The figure shows three views and two pictorial views of one solid part (mm, origin at its lowest corner). Answer the questions. Round coordinates to 2 decimals unless told otherwise and drop trailing zeros. Write each loop counter-clockwise with the first axis right and the second up, starting at its lowest first coordinate (ties: lowest second). Pieces come first, ordered by that corner, then holes. Notation, with made-up numbers: M 15.25,24 L 45.25,24 A11 cw 45.25,45 Z; hole C -17.75,6 d11. An arc over 180 degrees is marked long. One line per item, written item: value. Start each with the question number.
Q1. Consider probe 1 along X at (y, z) = (2.75, 5); probe 2 along Y at (x, z) = (22, 2.75); probe 3 along X at (y, z) = (20.25, 8.25). Determine where each line is inside the solid, lowest interval first.
Q2. The mould has two halves that part along Y. Classify the marked faces 1, 2 and 3: released by +Y, released by -Y, zero draft, split by the parting line, or undercut.
Q3. Find section D-D (x = 8). Write down the section's boundary in (y, z).
Q4. Find section B-B (y = 16.5). Write down the section's boundary in (x, z), and give its area (3 significant figures).
Q5. Find section C-C (z = 1.25). Write down the section's boundary in (x, y), and give its area (3 significant figures).
Q6. Given pin 1 Ø1.5 at (x, z) = (7.5, 6) entering from -Y, flat-ended and moving along its own axis, determine where the tip first touches the part or whether it passes through.
Q7. Find section A-A (x = 75.98). Write down the section's boundary in (y, z), and give its area (3 significant figures).
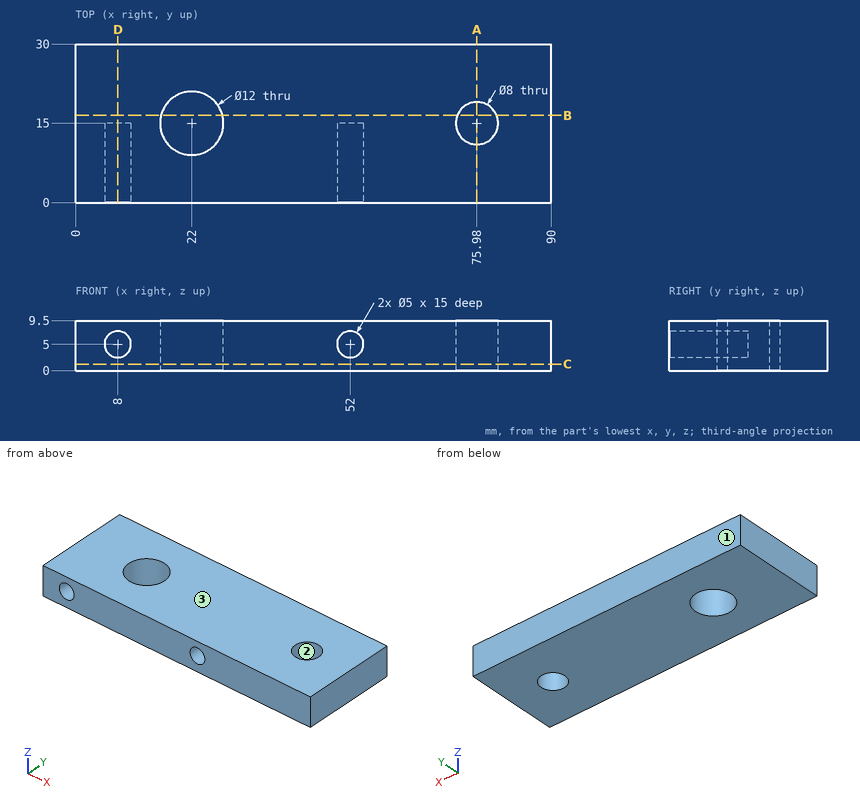
The answers:
1. probe 1: 0 to 5.5, 10.5 to 49.5, 54.5 to 90
1. probe 2: 0 to 9, 21 to 30
1. probe 3: 0 to 19.1, 24.9 to 90
2. face 1: released by +Y
2. face 2: undercut
2. face 3: zero draft
3. outline: M 0,0 L 30,0 L 30,9.5 L 0,9.5 L 0,7.5 L 15,7.5 L 15,2.5 L 0,2.5 Z
4. outline: M 0,0 L 16.19,0 L 16.19,9.5 L 0,9.5 Z; M 27.81,0 L 72.27,0 L 72.27,9.5 L 27.81,9.5 Z; M 79.69,0 L 90,0 L 90,9.5 L 79.69,9.5 Z
4. area: 674 mm2
5. outline: M 0,0 L 90,0 L 90,30 L 0,30 Z; hole C 22,15 d12; hole C 75.98,15 d8
5. area: 2,540 mm2
6. pin 1: y = 15
7. outline: M 0,0 L 11,0 L 11,9.5 L 0,9.5 Z; M 19,0 L 30,0 L 30,9.5 L 19,9.5 Z
7. area: 209 mm2
